```python
from build123d import *

# Parameters (mm, degrees)
SKETCH_2_R          = 1.55
CUT_EXTRUDE_1_DEPTH = 4
CUT_EXTRUDE_START   = -1.2
SKETCH_3_W          = 4
SKETCH_3_H          = 0.5
CUT_EXTRUDE_2_DEPTH = 1.2
CHAMFER_1_SIZE      = 0.2
CHAMFER_2_SIZE      = 0.1


with BuildPart() as part:
    # 草图1 → 旋转1 (revolve)
    with BuildSketch(Plane.XY, mode=Mode.PRIVATE) as revolve_1_sk:
        Polygon((-21.3, 0), (-21.3, 0.55), (-20.3, 0.55), (-20.3, 1.11), (-23.3, 1.11), (-24.65, -0.24), (-24.65, -0.89), (-24.5, -1.04), (-24.5, -1.69), (-24.65, -1.84), (-24.65, -2.19), (-24.5, -2.34), (-24.5, -2.69), (-24.65, -2.84), (-24.65, -3.19), (-24.5, -3.34), (-24.5, -3.69), (-24.65, -3.84), (-24.65, -8.435), (-21.3, -8.435), (-21.3, -3.615), (-22.3, -2.615), (-22.3, -1), align=None)
    revolve(revolve_1_sk.sketch.rotate(Axis((0, 0.266506915, 0), (0, 1, 0)), 270), axis=Axis((0, 0.266506915, 0), (0, 1, 0)))

    # 草图2 → 切除-拉伸1 (cut)
    with BuildSketch(Plane.XZ.offset(8.435)):
        with Locations(Location((19.875283017, 11.475, 0), (0, 0, 270))):
            Circle(SKETCH_2_R)
        with Locations(Location((19.875283017, -11.475, 0), (0, 0, 90))):
            Circle(SKETCH_2_R)
        with Locations(Location((-19.875283017, -11.475, 0), (0, 0, 270))):
            Circle(SKETCH_2_R)
        with Locations(Location((-19.875283017, 11.475, 0), (0, 0, 90))):
            Circle(SKETCH_2_R)
        with Locations(Location((0, 22.95, 0), (0, 0, 270))):
            Circle(SKETCH_2_R)
        with Locations(Location((0, -22.95, 0), (0, 0, 270))):
            Circle(SKETCH_2_R)
    extrude(amount=-CUT_EXTRUDE_1_DEPTH, mode=Mode.SUBTRACT)

    # 草图3 → 切除-拉伸2 (cut)
    with BuildSketch(Plane.XZ.offset(8.435).offset(CUT_EXTRUDE_START)):
        with BuildLine():
            Line((-16.757915815, 15.088895173), (-15.828984783, 14.252481915))
            ThreePointArc((-15.828984783, 14.252481915), (-10.65, 18.446341101), (-4.428519014, 20.834543896))
            Line((-4.428519014, 20.834543896), (-4.688408628, 22.057228397))
            ThreePointArc((-4.688408628, 22.057228397), (-11.275, 19.528872855), (-16.757915815, 15.088895173))
        make_face()
        with BuildLine():
            Line((4.688408628, 22.057228397), (4.428519014, 20.834543896))
            ThreePointArc((4.428519014, 20.834543896), (10.65, 18.446341101), (15.828984783, 14.252481915))
            Line((15.828984783, 14.252481915), (16.757915815, 15.088895173))
            ThreePointArc((16.757915815, 15.088895173), (11.275, 19.528872855), (4.688408628, 22.057228397))
        make_face()
        with BuildLine():
            Line((16.757915815, -15.088895173), (15.828984783, -14.252481915))
            ThreePointArc((15.828984783, -14.252481915), (10.65, -18.446341101), (4.428519014, -20.834543896))
            Line((4.428519014, -20.834543896), (4.688408628, -22.057228397))
            ThreePointArc((4.688408628, -22.057228397), (11.275, -19.528872855), (16.757915815, -15.088895173))
        make_face()
        with BuildLine():
            Line((21.446324442, 6.968333223), (20.257503797, 6.58206198))
            ThreePointArc((20.257503797, 6.58206198), (21.3, 0), (20.257503797, -6.58206198))
            Line((20.257503797, -6.58206198), (21.446324442, -6.968333223))
            ThreePointArc((21.446324442, -6.968333223), (22.55, 0), (21.446324442, 6.968333223))
        make_face()
        with BuildLine():
            Line((-21.446324442, -6.968333223), (-20.257503797, -6.58206198))
            ThreePointArc((-20.257503797, -6.58206198), (-21.3, 0), (-20.257503797, 6.58206198))
            Line((-20.257503797, 6.58206198), (-21.446324442, 6.968333223))
            ThreePointArc((-21.446324442, 6.968333223), (-22.55, 0), (-21.446324442, -6.968333223))
        make_face()
        with BuildLine():
            Line((-4.688408628, -22.057228397), (-4.428519014, -20.834543896))
            ThreePointArc((-4.428519014, -20.834543896), (-10.65, -18.446341101), (-15.828984783, -14.252481915))
            Line((-15.828984783, -14.252481915), (-16.757915815, -15.088895173))
            ThreePointArc((-16.757915815, -15.088895173), (-11.275, -19.528872855), (-4.688408628, -22.057228397))
        make_face()
        with Locations((0, -22.95)):
            Rectangle(SKETCH_3_W, SKETCH_3_H)
    extrude(amount=CUT_EXTRUDE_2_DEPTH, mode=Mode.SUBTRACT)

    # 倒角1
    chamfer_1_edges = [part.edges().sort_by_distance(p)[0] for p in [
        (-20.257503797, -7.835, 6.58206198),
        (-20.257503797, -7.835, -6.58206198),
        (20.257503797, -7.835, -6.58206198),
        (20.257503797, -7.835, 6.58206198),
        (4.428519014, -7.835, -20.834543896),
        (15.828984783, -7.835, -14.252481915),
        (15.828984783, -7.835, 14.252481915),
        (4.428519014, -7.835, 20.834543896),
        (-15.828984783, -7.835, -14.252481915),
        (-4.428519014, -7.835, -20.834543896),
        (-4.428519014, -7.835, 20.834543896),
        (-15.828984783, -7.835, 14.252481915),
    ]]
    chamfer(chamfer_1_edges, length=CHAMFER_1_SIZE)

    # 倒角2
    chamfer_2_edges = [part.edges().sort_by_distance(p)[0] for p in [
        (0, -8.435, 24.65),
    ]]
    chamfer(chamfer_2_edges, length=CHAMFER_2_SIZE)


solid = part.part
```
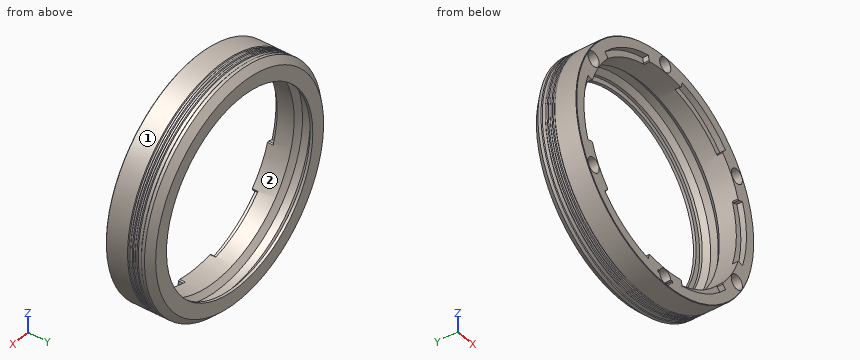
Could you check a few things on this model? Use its own coordinates, in mm. Face numbers are marked on the shaded views. A direction names the side the tool comes from. Round coordinates to 2 decimals unless told otherwise and drop trailing zeros. Loops run counter-clockwise (first coordinate to the right, second up) from the corner with the lowest first, then second, coordinate; pieces in that order, holes last. Notation, with made-up numbers: (43.5, -20) - (88.5, -20) arc R17 ccw to (88.5, 2) - close; hole circle Ø11 at (61, 24.25). An arc over 180 degrees is marked (long way). Use CSV: the item, a comma, the result in double quotes.
Item 1: Will these pins go through, and if not, where does the flat tip stop? pin 1 (2.5 mm diameter, centred on x = 0, z = -22.95, fed in from -Y) (3 decimals); pin 2 (4 mm diameter, centred on x = -9, z = -16.5, fed in from -Y); pin 3 (1 mm diameter, centred on y = -5.5, z = 4.5, fed in from -X).
Here are the results:
pin 1,"stops at y = -4.435"
pin 2,"stops at y = 0.55"
pin 3,"stops at x = -24.32"
Item 2: I need wall thicknesses on L1, parallel to Z at x = -19.5, y = -6; L2, parallel to Z at x = -5, y = -1.5; L3, parallel to X at y = -3.75, z = -3.5. Which ranges of each line are inside material? Lowest first, please. Write a range as [from, to].
Here are the results:
L1,"z = [-15.08, -12.98], [-9.97, -8.57], [8.57, 9.97], [12.98, 15.08]"
L2,"z = [-23.98, -21.73], [21.73, 23.98]"
L3,"x = [-24.31, -21.01], [21.01, 24.31]"
Item 3: For the marked faces 1 and 2, which set-ups out of +Z, -Z, +X, -X, +Y, -Y let a thin tool reach every point of the face, with its end or its side?
Here are the results:
face 1,"+Y, -Y"
face 2,"-Y"
Item 4: If we section it at A-A on y = -5.5: List the corners of the cut face in (x, z) for me (3 decimals), then the cut area to 3 significant figures.
Here are the results:
outline,"circle Ø49.3 at (0, 0); hole circle Ø3.1 at (-19.875, -11.475); hole circle Ø3.1 at (-19.875, 11.475); hole circle Ø42.6 at (0, 0); hole circle Ø3.1 at (0, -22.95); hole circle Ø3.1 at (0, 22.95); hole circle Ø3.1 at (19.875, -11.475); hole circle Ø3.1 at (19.875, 11.475)"
area,"438 mm²"
